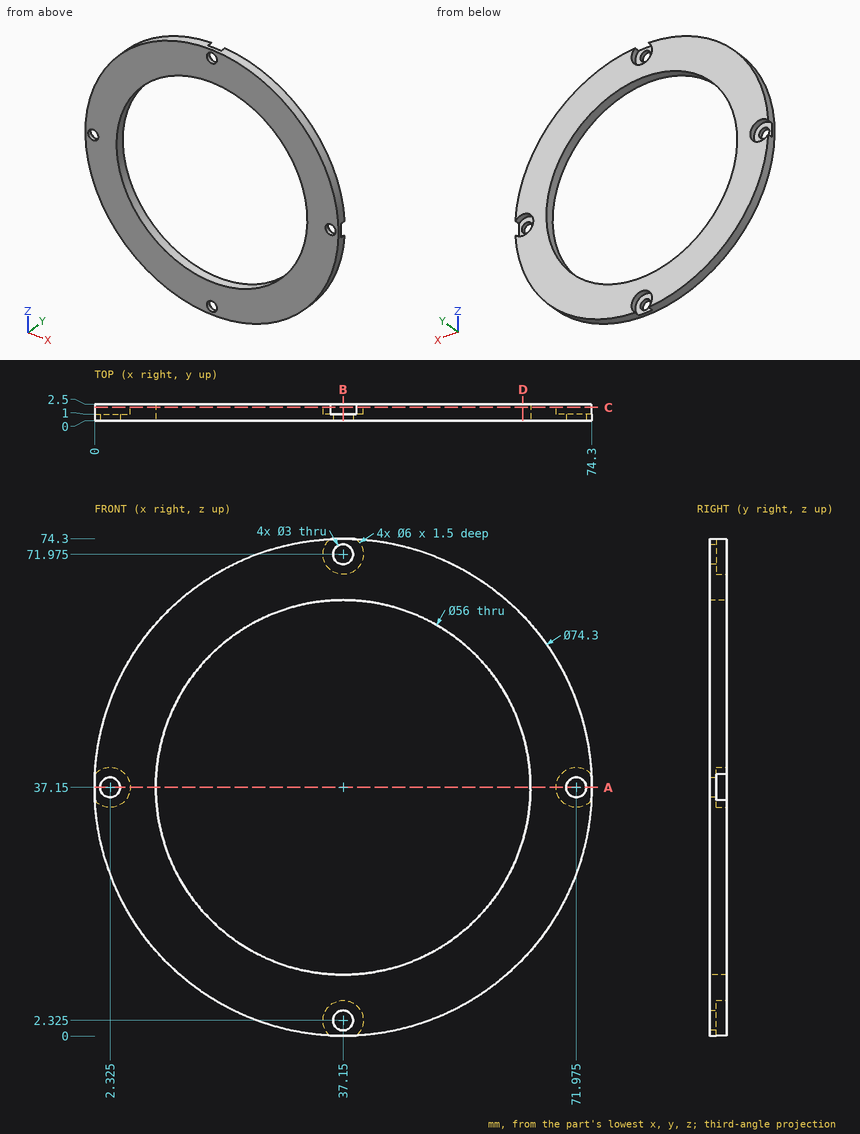
Job drawing, mm, ordinate dimensions from the low corner. One solid piece. Give positions to 0.01 mm unless a question says otherwise; leave off trailing zeros. Loops run counter-clockwise (first coordinate to the right, second up) from the corner with the lowest first, then second, coordinate; pieces in that order, holes last. Notation, with made-up numbers: M 64,-25.5 L 91,-25.5 A24 cw 91,-1.5 Z; hole C 69.5,-31 d9. An arc over 180 degrees is marked long. Put each result on its own line as item: value. Start each with the question number.
1) Saw through at D-D (x = 64). List the corners of the cut face in (y, z), then the cut area to 3 significant figures.
2) Saw through at C-C (y = 2). List the corners of the cut face in (x, z) (3 decimals), then the cut area to 3 significant figures.
3) Probe probe 1 along X at (y, z) = (0.7, 37.15) (3 decimals); probe 2 along Z at (x, y) = (37.15, 1.45) (3 decimals); probe 3 along Z at (x, y) = (36, 0.9). List the from-to ranges inside material, lowest first.
4) Saw through at B-B (x = 37.15). List the corners of the cut face in (y, z) (3 decimals), then the cut area to 3 significant figures.
5) Saw through at A-A (z = 37.15). List the corners of the cut face in (x, y) (3 decimals).
6) Flat gauge pins, fed straight in: pin 1 (1 mm diameter, centred on x = 17, y = 0.5, fed in from -Z); pin 2 (3.5 mm diameter, centred on x = 37.15, z = 2.325, fed in from +Y); pin 3 (1 mm diameter, centred on x = 61.5, y = 1, fed in from +Z). Where does each tip first touch, or does it go through?
Numbers:
1. outline: M 0,11.48 L 2.5,11.48 L 2.5,29.21 L 0,29.21 Z; M 0,45.09 L 2.5,45.09 L 2.5,62.82 L 0,62.82 Z
1. area: 88.7 mm^2
2. outline: M 0.052,35.193 A37.15 ccw 35.193,0.052 A3 cw long 39.107,0.052 A37.15 ccw 74.248,35.193 A3 cw long 74.248,39.107 A37.15 ccw 39.107,74.248 A3 cw long 35.193,74.248 A37.15 ccw 0.052,39.107 A3 cw long Z; hole C 37.15,37.15 d56
2. area: 1,770 mm^2
3. probe 1: 0 to 0.825, 3.825 to 9.15, 65.15 to 70.475, 73.475 to 74.3
3. probe 2: 5.325 to 9.15, 65.15 to 68.975
3. probe 3: 0.02 to 1.36, 3.29 to 9.17, 65.13 to 71.01, 72.94 to 74.28
4. outline: M 0,0 L 1,0 L 1,0.825 L 0,0.825 Z; M 0,3.825 L 1,3.825 L 1,5.325 L 2.5,5.325 L 2.5,9.15 L 0,9.15 Z; M 0,65.15 L 2.5,65.15 L 2.5,68.975 L 1,68.975 L 1,70.475 L 0,70.475 Z; M 0,73.475 L 1,73.475 L 1,74.3 L 0,74.3 Z
4. area: 23.8 mm^2
5. outline: M 0,0 L 0.825,0 L 0.825,1 L 0,1 Z; M 3.825,0 L 9.15,0 L 9.15,2.5 L 5.325,2.5 L 5.325,1 L 3.825,1 Z; M 65.15,0 L 70.475,0 L 70.475,1 L 68.975,1 L 68.975,2.5 L 65.15,2.5 Z; M 73.475,0 L 74.3,0 L 74.3,1 L 73.475,1 Z
6. pin 1: z = 5.62
6. pin 2: y = 1
6. pin 3: z = 65.63
